Verification items for the finished model (mm, model axes). Face numbers are marked on the shaded views. A direction names the side the tool comes from. Round coordinates to 2 decimals unless told otherwise and drop trailing zeros. Loops run counter-clockwise (first coordinate to the right, second up) from the corner with the lowest first, then second, coordinate; pieces in that order, holes last. Notation, with made-up numbers: M -6,48 L 11,48 A27 cw 11,79 Z; hole C -36.75,-13 d4. An arc over 180 degrees is marked long. One line per item, written item: value.
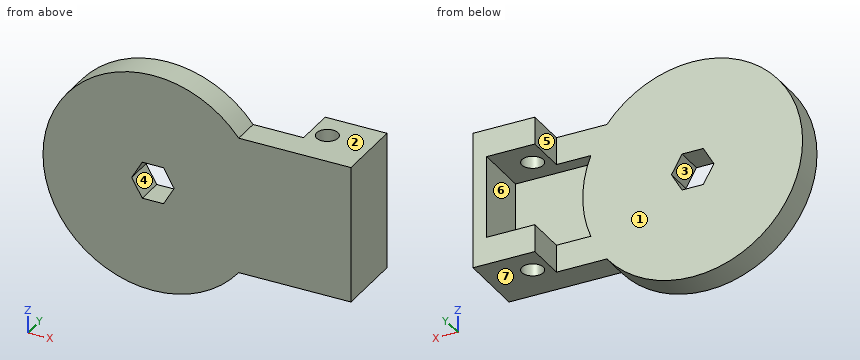
Autodesk Inventor part; units mm, degrees
ref_plane "YZ Plane" through (0, 0, 0) normal (1, 0, 0) x (0, 1, 0)
ref_plane "XZ Plane" through (0, 0, 0) normal (0, 1, 0) x (-1, 0, 0)
ref_plane "XY Plane" through (0, 0, 0) normal (0, 0, 1) x (1, 0, 0)
sketch "Sketch1" plane through (0, 0, 0) normal (0, 0, 1) x (1, 0, 0)
  line L0 (0, 0) -> (-50.8, 0)
  line L1 (-50.8, 0) -> (-50.8, -12.7)
  line L2 (-50.8, -12.7) -> (-38.1, -12.7)
  line L3 (-12.0663, -25.4) -> (-12.0663, -48.26)
  line L4 (-5, -48.26) -> (-5, -16.764)
  line L5 (-5, -16.764) -> (0, -16.764)
  line L6 (0, -16.764) -> (0, 0)
  line L7 (-12.0663, -48.26) -> (-5, -48.26)
  line L8 (-38.1, -12.7) -> (-38.1, -25.4)
  line L9 (-38.1, -25.4) -> (-12.0663, -25.4)
  dimension "d0" = 50.8
  dimension "d1" = 5
  dimension "d2" = 12.0663
  dimension "d13" = 35.56
  dimension "d15" = 31.496
  dimension "d38" = 12.7
  dimension "d39" = 38.1
revolve "Revolution1" add sketch "Sketch1" angle 360 about axis through (0, -16.764, 0) along (0, 1, 0)
sketch "Sketch5" plane through (0, 0, 0) normal (0, 1, 0) x (1, 0, 0)
  circle A0 centre (0, 0) radius 5
  line L0 (9.815, 0) -> (4.9075, -8.5)
  line L1 (4.9075, -8.5) -> (-4.9075, -8.5)
  line L2 (-4.9075, -8.5) -> (-9.815, 0)
  line L3 (-9.815, 0) -> (-4.9075, 8.5)
  line L4 (-4.9075, 8.5) -> (4.9075, 8.5)
  line L5 (4.9075, 8.5) -> (9.815, 0)
  point P0 (0, 0)
  point P1 (0, 0)
  dimension "d16" = 17
extrude "Extrusion1" cut sketch "Sketch5" against normal blind 12.7 contours A0 | L0 L1 L2 L3 L4 L5
sketch "Sketch7" plane through (0, -12.7, 0) normal (0, -1, 0) x (1, 0, 0)
  circle A0 centre (0, 0) radius 50.8
  line L0 (47.0929, -19.05) -> (85.1929, -19.05)
  line L1 (85.1929, -19.05) -> (85.1929, -31.75)
  line L2 (85.1929, -31.75) -> (39.6557, -31.75)
  circle A1 centre (0, 0) radius 5 construction
  line L3 (0, 0) -> (5, 0) construction
  line L4 (50.8, 0) -> (83.823, 0) construction
  dimension "d23" = 38.1
  dimension "d24" = 12.7
  dimension "d25" = 19.05
extrude "Extrusion3" add sketch "Sketch7" against normal blind 12.7 contours A0 L0 L1 L2
sketch "Sketch8" plane through (39.6557, 0, -31.75) normal (0, 1, 0) x (1, 0, 0)
  line L0 (45.5371, -12.7) -> (45.5371, 0)
  line L1 (45.5371, 0) -> (0, 0)
  line L2 (7.4371, -12.7) -> (45.5371, -12.7)
  line L3 (35.8511, -107.95) -> (35.8511, 44.45)
  line L4 (26.3261, -107.95) -> (26.3261, 44.45)
  line L5 (45.5371, -12.7) -> (23.3121, -12.7)
  line L6 (23.3121, -12.7) -> (23.3121, 0)
  line L7 (23.3121, 0) -> (45.5371, 0)
  line L8 (45.5371, 0) -> (45.5371, -12.7)
  point P0 (-39.6557, -31.75)
  point P1 (23.3121, 0)
  point P2 (23.3121, -12.7)
  dimension "d28" = 22.225
extrude "Extrusion4" add sketch "Sketch8" along normal blind 19.05
sketch "Sketch9" plane through (85.1929, -12.7, -31.75) normal (0, 0, -1) x (-1, 0, 0)
  line L0 (22.225, 12.7) -> (22.225, 31.75)
  line L1 (0, 31.75) -> (22.225, 31.75)
  arc A0 (16.0423, 14.3621) -> (12.8546, 14.3621) centre (14.4485, 18.85) ccw
  line L2 (0, 0) -> (0, 31.75)
  circle A1 centre (14.4485, 18.85) radius 4.953
  point P0 (85.1929, 12.7)
  dimension "d31" = 9.906
extrude "Extrusion5" cut sketch "Sketch9" against normal through all
mirror "Mirror1" about plane through (0, 0, 0) normal (0, 0, 1) of "Extrusion4", "Extrusion5", "Extrusion3"
sketch "Sketch10" plane through (39.6557, -12.7, -31.75) normal (0, -1, 0) x (1, 0, 0)
  arc A0 (7.4371, 12.7) -> (7.4371, 50.8) centre (-39.6557, 31.75) ccw
  line L0 (45.5371, 50.8) -> (7.4371, 50.8)
  line L1 (45.5371, 12.7) -> (7.4371, 12.7)
  arc A1 (7.4371, 12.7) -> (7.4371, 50.8) centre (-39.6557, 31.75) ccw
  line L2 (7.4371, 50.8) -> (45.5371, 50.8)
  line L3 (45.5371, 0) -> (45.5371, 12.7)
  line L4 (45.5371, 50.8) -> (45.5371, 12.7)
  line L5 (45.5371, 12.7) -> (7.4371, 12.7)
extrude "Extrusion6" add sketch "Sketch10" against normal blind 6.35
sketch "Sketch11" plane through (85.1929, -12.7, -31.75) normal (1, 0, 0) x (0, 0, -1)
  line L0 (-63.5, 0) -> (-63.5, 31.75)
  line L1 (-50.8, 31.75) -> (-63.5, 31.75)
  line L2 (-12.7, 31.75) -> (0, 31.75)
  line L3 (0, 0) -> (0, 31.75)
  line L4 (0, 0) -> (-63.5, 0)
  line L5 (-63.5, 31.75) -> (0, 31.75)
  line L6 (0, 31.75) -> (0, 0)
  line L7 (0, 0) -> (-63.5, 0)
  line L8 (-63.5, 0) -> (-63.5, 31.75)
  point P0 (-31.75, 12.7)
  point P1 (-12.7, 31.75)
  point P2 (-50.8, 31.75)
extrude "Extrusion7" add sketch "Sketch11" along normal blind 6.35
sketch "Sketch13" plane through (0, -12.7, 0) normal (0, -1, 0) x (1, 0, 0)
  circle A0 centre (0, 0) radius 38.1
extrude "Extrusion8" cut sketch "Sketch13" along normal through all
equation "\"d0\" = topPartRadius"
equation "\"d2\" = stemRadius"
equation "\"d15\" = internalHoleDepth"
equation "\"topPartRadius\" = 0.5 * topPartDiameter"
equation "\"totalHeight\" = 35.56"
equation "\"stemRadius\" = 12.06627"
equation "\"stemHeight\" = 22.86"
equation "\"internalHoleDepth\" = 31.496"
equation "\"topPartDiameter\" = 101.6"
properties part number "celestronTripodAdapterTop" material "PC/ABS Plastic"
(1) Sectioned sample at B-B on y = 6.15. Enter the section's corners in (x, z), and give its area (3 significant figures).
Completed:
outline: M 62.97,-31.75 L 65.79,-31.75 L 65.79,-19.05 L 62.97,-19.05 Z; M 62.97,19.05 L 65.79,19.05 L 65.79,31.75 L 62.97,31.75 Z; M 75.7,-31.75 L 91.54,-31.75 L 91.54,31.75 L 75.7,31.75 L 75.7,19.05 L 85.19,19.05 L 85.19,-19.05 L 75.7,-19.05 Z
area: 716 mm^2
(2) Tool access check on the marked faces 4, 5, 6 and 7. Record the directions out of +Z, -Z, +X, -X, +Y, -Y that give a thin tool (end or side, any length) a straight path to the whole face; none if there is none.
Completed:
face 4: +Y, -Y
face 5: +Z, -Z, -X, +Y
face 6: +Y
face 7: -Z, +X, +Y, -Y
(3) Thickness scan on L1, parallel to X at y = 6, z = 23; L2, parallel to Z at x = 77.5, y = 3; L3, parallel to Y at x = -36, z = -8.5. Record the ranges inside material, lowest first. Write a range as from..to.
Completed:
L1: x = 62.97..65.79, 75.7..91.54
L2: z = -31.75..-19.05, 19.05..31.75
L3: y = -12.7..0
(4) Mould release check, pull along Z, two halves, no side actions. Record for the marked faces 1, 2 and 3: +Z half, -Z half, draft (parallel to the pull), parting line (faces both ways), or undercut.
Completed:
face 1: draft
face 2: +Z half
face 3: undercut
(5) Sectioned sample at A-A on x = 0. Enter the section's corners in (y, z).
Completed:
outline: M -12.7,-50.8 L 0,-50.8 L 0,-8.5 L -12.7,-8.5 Z; M -12.7,8.5 L 0,8.5 L 0,50.8 L -12.7,50.8 Z
(6) Sectioned sample at C-C on z = -25. Enter the section's corners in (x, y), and give its area (3 significant figures).
Completed:
outline: M -44.22,-12.7 L 91.54,-12.7 L 91.54,19.05 L 62.97,19.05 L 62.97,0 L -44.22,0 Z; hole C 70.74,6.15 d9.91
area: 2,190 mm^2
(7) Sectioned sample at D-D on z = -3. Enter the section's corners in (x, y).
Completed:
outline: M -50.71,-12.7 L -8.08,-12.7 L -8.08,0 L -50.71,0 Z; M 8.08,-12.7 L 91.54,-12.7 L 91.54,19.05 L 85.19,19.05 L 85.19,-6.35 L 50.71,-6.35 L 50.71,0 L 8.08,0 Z
(8) Depth check by flat-ended pin: pin 1 Ø7.5 at (x, y) = (72, 9) entering from +Z; pin 2 Ø1.5 at (x, y) = (13, -6) entering from -Z; pin 3 Ø2 at (x, y) = (-18, -7.5) entering from +Z; pin 4 Ø9 at (x, y) = (70.74, 6.15) entering from +Z. Enter the tip coordinate at first touch or a pass-through.
Completed:
pin 1: stops at z = 31.75
pin 2: stops at z = -49.3
pin 3: stops at z = 47.87
pin 4: passes through
